Verification items for the finished model (mm, model axes). A direction names the side the tool comes from. Round coordinates to 2 decimals unless told otherwise and drop trailing zeros. Write each loop counter-clockwise with the first axis right and the second up, starting at its lowest first coordinate (ties: lowest second). Pieces come first, ordered by that corner, then holes.
from build123d import *

# Parameters (mm, degrees)
CUT_EXTRUDE_2_REACH = 10.967
SKETCH_5_W          = 0.5
SKETCH_5_H          = 0.5
EXTRUDE_1_DEPTH     = 3


with BuildPart() as part:
    # Эскиз1 → Повернуть1 (revolve)
    with BuildSketch(Plane(origin=(0, 0, 0), x_dir=(0, 0, -1), z_dir=(1, 0, 0)), mode=Mode.PRIVATE) as revolve_1_sk:
        with BuildLine():
            Line((-2.5, 1), (0, 1))
            Line((0, 1), (0, 8.7))
            ThreePointArc((0, 8.7), (-1.767766953, 7.967766953), (-2.5, 6.2))
            Line((-2.5, 6.2), (-2.5, 1))
        make_face()
        Polygon((-3.25, 1), (-3.25, 0), (0, 0), (0, 1), (-2.5, 1), align=None)
    revolve(revolve_1_sk.sketch.rotate(Axis((0, -2.603301624, 0), (0, 1, 0)), 180), axis=Axis((0, -2.603301624, 0), (0, 1, 0)))

    # Эскиз4 → Вырез-Вытянуть2 (cut, up to next)
    with BuildSketch(Plane(origin=(0, 1, 0), x_dir=(1, 0, 0), z_dir=(0, 1, 0)), mode=Mode.PRIVATE) as cut_extrude_2_sk1:
        with BuildLine():
            Line((-2.5, 2.076655966), (-2.5, -2.076655966))
            ThreePointArc((-2.5, -2.076655966), (-3.25, 0), (-2.5, 2.076655966))
        make_face()
    cut_extrude_2_tool1 = extrude(cut_extrude_2_sk1.sketch, amount=-CUT_EXTRUDE_2_REACH, mode=Mode.PRIVATE) & part.part
    add(cut_extrude_2_tool1.solids().sort_by_distance((-2.80318, 1, 0))[0], mode=Mode.SUBTRACT)

    # Эскиз5 → Бобышка-Вытянуть1 (add)
    with BuildSketch(Plane.XZ):
        with Locations((0, 0.7)):
            Rectangle(SKETCH_5_W, SKETCH_5_H)
        with Locations((0, 2.1)):
            Rectangle(SKETCH_5_W, SKETCH_5_H)
        with Locations((0, -0.7)):
            Rectangle(SKETCH_5_W, SKETCH_5_H)
        with Locations((0, -2.1)):
            Rectangle(SKETCH_5_W, SKETCH_5_H)
    extrude(amount=EXTRUDE_1_DEPTH)


solid = part.part
Q1. Tool access check on faces 1 (the cylindrical face through (-0.1, 3.6, 2.5)), 2 (the flat face through (-2.5, 0.5, 0)). Record the directions out of +Z, -Z, +X, -X, +Y, -Y that give a thin tool (end or side, any length) a straight path to the whole face; none if there is none.
Recorded:
face 1: +Y
face 2: +Z, -Z, -X, +Y, -Y
Q2. Depth check by flat-ended pin: P1, Ø1, axis at x = 2.5, z = 2.5, coming from the +Y side; P2, Ø0.6, axis at x = 0, y = -2, coming from the -Z side; P3, Ø2, axis at y = 2.5, z = -2.5, coming from the -X side. Enter the tip coordinate at first touch or a pass-through.
Recorded:
P1: stops at y = 1
P2: stops at z = -2.35
P3: stops at x = -2
Q3. Sectioned sample at B-B (y = -0.25). Enter the section's corners in (x, z).
Recorded:
outline: (-0.25, -2.35) - (0.25, -2.35) - (0.25, -1.85) - (-0.25, -1.85) - close; (-0.25, -0.95) - (0.25, -0.95) - (0.25, -0.45) - (-0.25, -0.45) - close; (-0.25, 0.45) - (0.25, 0.45) - (0.25, 0.95) - (-0.25, 0.95) - close; (-0.25, 1.85) - (0.25, 1.85) - (0.25, 2.35) - (-0.25, 2.35) - close
Q4. Sectioned sample at D-D (y = 4). Enter the section's corners in (x, z).
Recorded:
outline: circle Ø5 at (0, 0)
Q5. Sectioned sample at A-A (x = 0). Enter the section's corners in (y, z).
Recorded:
outline: (-3, -2.35) - (0, -2.35) - (0, -3.25) - (1, -3.25) - (1, -2.5) - (6.2, -2.5) arc R2.5 ccw to (6.2, 2.5) - (1, 2.5) - (1, 3.25) - (0, 3.25) - (0, 2.35) - (-3, 2.35) - (-3, 1.85) - (0, 1.85) - (0, 0.95) - (-3, 0.95) - (-3, 0.45) - (0, 0.45) - (0, -0.45) - (-3, -0.45) - (-3, -0.95) - (0, -0.95) - (0, -1.85) - (-3, -1.85) - close
Q6. Material ranges on line 1 along Y through (x, z) = (0.7, -2.5); line 2 along X through (y, z) = (-0.75, 0.5); line 3 along Z through (x, y) = (-1.55, 4), recorded low to high.
Recorded:
line 1: y = 0 to 1
line 2: x = -0.25 to 0.25
line 3: z = -1.96 to 1.96
